Design review of the part built by this model. Coordinates are the model's own, in mm. Face numbers are marked on the shaded views. A direction names the side the tool comes from. Give positions to 0.01 mm unless a question says otherwise; leave off trailing zeros. Loops run counter-clockwise (first coordinate to the right, second up) from the corner with the lowest first, then second, coordinate; pieces in that order, holes last. Notation, with made-up numbers: M -32.75,38 L -20.75,38 A15 ccw -20.75,66 Z; hole C 88.5,71.25 d5. An arc over 180 degrees is marked long. Use a Markdown table: item, result. Add a question column.
(1) Add section A-A, the plane y = 5. State how many separate pieces and enclosed holes the cut face has, then the cut area to 3 significant figures.
(2) For the marked faces 1, 2 and 3, list the 3-axis set-ups (+Z, -Z, +X, -X, +Y, -Y) from which the entire face can be reached by the end or side of a thin tool; tool diameter is ignored.
(3) For probe 1 along Y at (x, z) = (17, 8.5); probe 2 along Y at (x, z) = (120, 5.5); probe 3 along Y at (x, z) = (10, 6.5), list the stretches that pass through material, from the lowest coordinate up.
(4) Add section D-D, the plane y = 16.5. Give the boundary of the cut face in (x, z).
(5) Insertion check: pin 1 Ø2 at (x, z) = (30, 6.5) entering from -Y; pin 2 Ø5.5 at (x, y) = (65, 60) entering from -Z; pin 3 Ø2.5 at (x, y) = (120, 5) entering from -Z; pin 4 Ø1 at (y, z) = (47.5, 8.5) entering from +X. Each pin has a flat end and moves straight along its axis. Give the tip position at first contact, or say it passes through.
(6) Draft analysis for pull direction Y (two halves, no side actions). For the marked faces 4, 5, 6 and 7, state which applies: pulls with the +Y half, pulls with the -Y half, needs draft (parallel to the pull), parting line crosses it, or undercut.
(7) Add section B-B, the plane x = 10. Give the boundary of the cut face in (y, z), then the cut area to 3 significant figures.
```python
from build123d import *

# Parameters (mm, degrees)
ESQUISSE1_W             = 130
ESQUISSE1_H             = 65
ESQUISSE1_R             = 1.3
BOSS_EXTRU_1_DEPTH      = 15
ESQUISSE2_W             = 130
ESQUISSE2_H             = 12.5
ESQUISSE2_H_2           = 22
ENL_V_MAT_EXTRU_1_DEPTH = 0.5
ESQUISSE5_R             = 1.3
ENL_V_MAT_EXTRU_2_DEPTH = 15.5
D_GAGEMENT_M31_D        = 3.4
ENL_V_MAT_EXTRU_3_DEPTH = 12
D_GAGEMENT_M61_D        = 6.6
D_GAGEMENT_M61_DEPTH    = 10
D_GAGEMENT_M61_TIP      = 1.982840043
ESQUISSE16_W            = 98
ESQUISSE16_H            = 1.5
ESQUISSE16_W_2          = 95
BOSS_EXTRU_2_DEPTH      = 12


with BuildPart() as part:
    # Esquisse1 → Boss.-Extru.1 (new body)
    with BuildSketch(Plane.XY):
        with Locations((65, 32.5)):
            Rectangle(ESQUISSE1_W, ESQUISSE1_H)
        with Locations((113, 5)):
            Circle(ESQUISSE1_R, mode=Mode.SUBTRACT)
        with Locations((89, 5)):
            Circle(ESQUISSE1_R, mode=Mode.SUBTRACT)
        with Locations((65, 5)):
            Circle(ESQUISSE1_R, mode=Mode.SUBTRACT)
        with Locations((41, 5)):
            Circle(ESQUISSE1_R, mode=Mode.SUBTRACT)
        with Locations((17, 5)):
            Circle(ESQUISSE1_R, mode=Mode.SUBTRACT)
        with Locations((113, 60)):
            Circle(ESQUISSE1_R, mode=Mode.SUBTRACT)
        with Locations((89, 60)):
            Circle(ESQUISSE1_R, mode=Mode.SUBTRACT)
        with Locations((65, 60)):
            Circle(ESQUISSE1_R, mode=Mode.SUBTRACT)
        with Locations((41, 60)):
            Circle(ESQUISSE1_R, mode=Mode.SUBTRACT)
        with Locations((17, 60)):
            Circle(ESQUISSE1_R, mode=Mode.SUBTRACT)
    extrude(amount=BOSS_EXTRU_1_DEPTH)

    # Esquisse2 → Enlèv. mat.-Extru.1 (cut)
    with BuildSketch(Plane(origin=(0, 0, 0), x_dir=(-1, 0, 0), z_dir=(0, 0, -1))):
        with Locations((-65, 58.75)):
            Rectangle(ESQUISSE2_W, ESQUISSE2_H)
        with Locations((-65, 6.25)):
            Rectangle(ESQUISSE2_W, ESQUISSE2_H)
        with Locations((-65, 32.5)):
            Rectangle(ESQUISSE2_W, ESQUISSE2_H_2)
    extrude(amount=-ENL_V_MAT_EXTRU_1_DEPTH, mode=Mode.SUBTRACT)

    # Esquisse5 → Enlèv. mat.-Extru.2 (cut, through all)
    with BuildSketch(Plane(origin=(0, 0, 0.5), x_dir=(-1, 0, 0), z_dir=(0, 0, -1))):
        with Locations((-95, 32.5)):
            Circle(ESQUISSE5_R)
        with Locations((-65, 32.5)):
            Circle(ESQUISSE5_R)
        with Locations((-125, 32.5)):
            Circle(ESQUISSE5_R)
        with Locations((-5, 32.5)):
            Circle(ESQUISSE5_R)
        with Locations((-10, 60)):
            Circle(ESQUISSE5_R)
        with Locations((-10, 5)):
            Circle(ESQUISSE5_R)
        with Locations((-120, 60)):
            Circle(ESQUISSE5_R)
        with Locations((-120, 5)):
            Circle(ESQUISSE5_R)
        with Locations((-35, 32.5)):
            Circle(ESQUISSE5_R)
    extrude(amount=-ENL_V_MAT_EXTRU_2_DEPTH, mode=Mode.SUBTRACT)

    # Dégagement M31 (through all)
    with Locations(Plane.XY.offset(15)):
        with Locations((17, 60), (41, 60), (65, 60), (89, 60), (113, 60), (125, 32.5), (95, 32.5), (65, 32.5), (5, 32.5), (17, 5), (41, 5), (65, 5), (89, 5), (113, 5), (10, 60), (10, 5), (120, 5), (120, 60), (35, 32.5)):
            Hole(D_GAGEMENT_M31_D / 2)

    # Esquisse12 → Enlèv. mat.-Extru.3 (cut)
    with BuildSketch(Plane.XY.offset(15)):
        with BuildLine():
            Line((122, 55), (17, 55))
            ThreePointArc((17, 55), (15.585786438, 54.414213562), (15, 53))
            Line((15, 53), (15, 12))
            ThreePointArc((15, 12), (15.585786438, 10.585786438), (17, 10))
            Line((17, 10), (122, 10))
            ThreePointArc((122, 10), (123.414213562, 10.585786438), (124, 12))
            Line((124, 12), (124, 21))
            ThreePointArc((124, 21), (123.414213562, 22.414213562), (122, 23))
            Line((122, 23), (22, 23))
            ThreePointArc((22, 23), (20.585786438, 23.585786438), (20, 25))
            Line((20, 25), (20, 40))
            ThreePointArc((20, 40), (20.585786438, 41.414213562), (22, 42))
            Line((22, 42), (122, 42))
            ThreePointArc((122, 42), (123.414213562, 42.585786438), (124, 44))
            Line((124, 44), (124, 53))
            ThreePointArc((124, 53), (123.414213562, 54.414213562), (122, 55))
        make_face()
    extrude(amount=-ENL_V_MAT_EXTRU_3_DEPTH, mode=Mode.SUBTRACT)

    # Dégagement M61
    with Locations(Plane(origin=(130, 0, 0), x_dir=(0, 0, -1), z_dir=(1, 0, 0))):
        with Locations((-8, 48.5), (-8, 16.5)):
            Hole(D_GAGEMENT_M61_D / 2, depth=D_GAGEMENT_M61_DEPTH)
            with Locations((0, 0, -(D_GAGEMENT_M61_DEPTH + D_GAGEMENT_M61_TIP / 2))):  # 118° drill point
                Cone(0, D_GAGEMENT_M61_D / 2, D_GAGEMENT_M61_TIP, mode=Mode.SUBTRACT)

    # Esquisse16 → Boss.-Extru.2 (add)
    with BuildSketch(Plane.XY.offset(3)):
        with Locations((69, 51.25)):
            Rectangle(ESQUISSE16_W, ESQUISSE16_H)
        with Locations((70.5, 45.75)):
            Rectangle(ESQUISSE16_W_2, ESQUISSE16_H)
        with Locations((70.5, 19.25)):
            Rectangle(ESQUISSE16_W_2, ESQUISSE16_H)
        with Locations((69, 13.75)):
            Rectangle(ESQUISSE16_W, ESQUISSE16_H)
    extrude(amount=BOSS_EXTRU_2_DEPTH)


solid = part.part
```
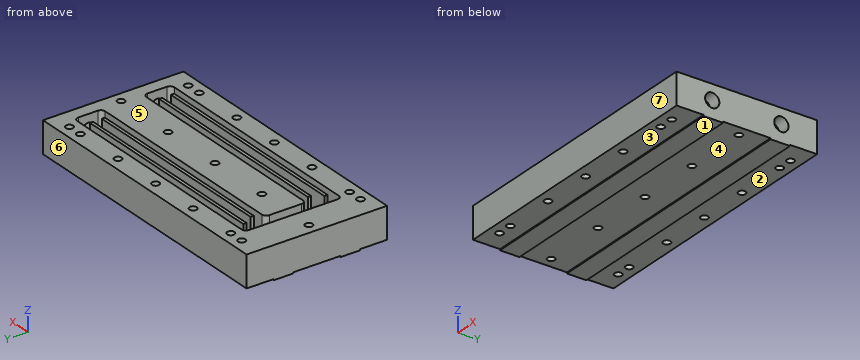
Established:
| question | item | result |
|---|---|---|
| 1 | separate pieces | 8 |
| 1 | enclosed holes | 0 |
| 1 | area | 1,540 mm^2 |
| 2 | face 1 | -Z, +X, -X, +Y, -Y |
| 2 | face 2 | -Z, +X, -X, +Y |
| 2 | face 3 | -Z, +X, -X, -Y |
| 3 | probe 1 | 0 to 3.3, 6.7 to 10, 55 to 58.3, 61.7 to 65 |
| 3 | probe 2 | 0 to 3.3, 6.7 to 10, 23 to 42, 55 to 58.3, 61.7 to 65 |
| 3 | probe 3 | 0 to 3.3, 6.7 to 58.3, 61.7 to 65 |
| 4 | outline | M 0,0 L 130,0 L 130,4.7 L 124,4.7 L 124,3 L 15,3 L 15,15 L 0,15 Z; M 124,11.3 L 130,11.3 L 130,15 L 124,15 Z |
| 5 | pin 1 | y = 0 |
| 5 | pin 2 | z = 0.5 |
| 5 | pin 3 | through |
| 5 | pin 4 | x = 15 |
| 6 | face 4 | undercut |
| 6 | face 5 | needs draft |
| 6 | face 6 | pulls with the +Y half |
| 6 | face 7 | pulls with the -Y half |
| 7 | outline | M 0,0.5 L 3.3,0.5 L 3.3,15 L 0,15 Z; M 6.7,0.5 L 12.5,0.5 L 12.5,0 L 21.5,0 L 21.5,0.5 L 43.5,0.5 L 43.5,0 L 52.5,0 L 52.5,0.5 L 58.3,0.5 L 58.3,15 L 6.7,15 Z; M 61.7,0.5 L 65,0.5 L 65,15 L 61.7,15 Z |
| 7 | area | 853 mm^2 |
